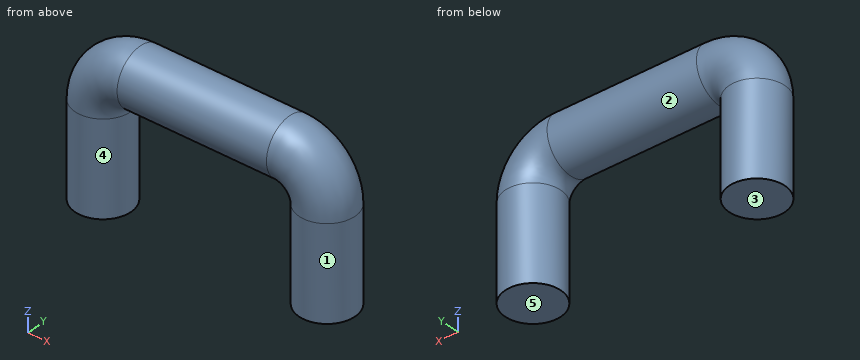
from build123d import *

# Parameters (mm, degrees)
F0_R = 1.5


with BuildPart() as f2:
    # F2: sweep along a path in F1
    with BuildLine(Plane.XZ) as f2_path:
        Line((-6, 0), (-6, 5))
        ThreePointArc((-6, 5), (-5.4142135624, 6.4142135624), (-4, 7))
        Line((-4, 7), (0, 7))
    # F0 (on Top) → F2 (sweep)
    with BuildSketch(Plane.XY):
        with Locations((-6, 0)):
            Circle(F0_R)
    sweep(path=f2_path.line)

    # F3: F2 across plane


with BuildPart() as f2_1:
    add(f2.part)
    add(f2.part.mirror(Plane.YZ))


solid = f2_1.part
Geometry check sheet. Reference: the model listing, model coordinates, mm. Face numbers are marked on the shaded views. A direction names the side the tool comes from. Give positions to 0.01 mm unless a question says otherwise; leave off trailing zeros. Loops run counter-clockwise (first coordinate to the right, second up) from the corner with the lowest first, then second, coordinate; pieces in that order, holes last. Notation, with made-up numbers: M -22.75,53.5 L 3.25,53.5 A22 cw 3.25,83.5 Z; hole C 69.25,-39.5 d8. An arc over 180 degrees is marked long. Answer as a JSON object with one key per item and string values. Group by question number.
Item 1: Sectioned sample at A-A on y = 0. Record the boundary of the cut face in (x, z), plus the area to 3 significant figures.
Item 2: Gauge pin test, flat ends, axial feed: pin 1 (1.5 mm diameter, centred on y = -1, z = 4, fed in from -X); pin 2 (1.5 mm diameter, centred on x = 4, z = 3.5, fed in from -Y). Record the tip position at first contact, or that the pin passes through.
Item 3: Access from +Z, -Z, +X, -X, +Y, -Y to the whole of each face (thin tool, end or side, straight path). Record for the marked faces 1, 2 and 3.
Item 4: Sectioned sample at C-C on z = 3.75. Record the boundary of the cut face in (x, y).
Item 5: Material ranges on L1, parallel to X at y = -0.6, z = 5; L2, parallel to X at y = 0.1, z = 4.5; L3, parallel to Y at x = -6.25, z = 7.5, recorded low to high.
Item 6: Mould release check, pull along X, two halves, no side actions. Record for the marked faces 4 and 5: pulls with the +X half, pulls with the -X half, needs draft (parallel to the pull), parting line crosses it, or undercut.
Item 7: Sectioned sample at B-B on x = -3.75. Record the boundary of the cut face in (y, z).
Findings below:
{
 "1": {"outline": "M -7.5,0 L -4.5,0 L -4.5,5 A0.5 cw -4,5.5 L 4,5.5 A0.5 cw 4.5,5 L 4.5,0 L 7.5,0 L 7.5,5 A3.5 ccw 4,8.5 L -4,8.5 A3.5 ccw -7.5,5 Z", "area": "72.8 mm2"},
 "2": {"pin 1": "x = -7.48", "pin 2": "y = -0.83"},
 "3": {"face 1": "-Z", "face 2": "none", "face 3": "-Z, +X, -X, +Y, -Y"},
 "4": {"outline": "C -6,0 d3; C 6,0 d3"},
 "5": {"L1": "-7.37 to -4.63, 4.63 to 7.37", "L2": "-7.5 to -4.5, 4.5 to 7.5", "L3": "-0.63 to 0.63"},
 "6": {"face 4": "undercut", "face 5": "needs draft"},
 "7": {"outline": "C 0,7 d3"}
}
